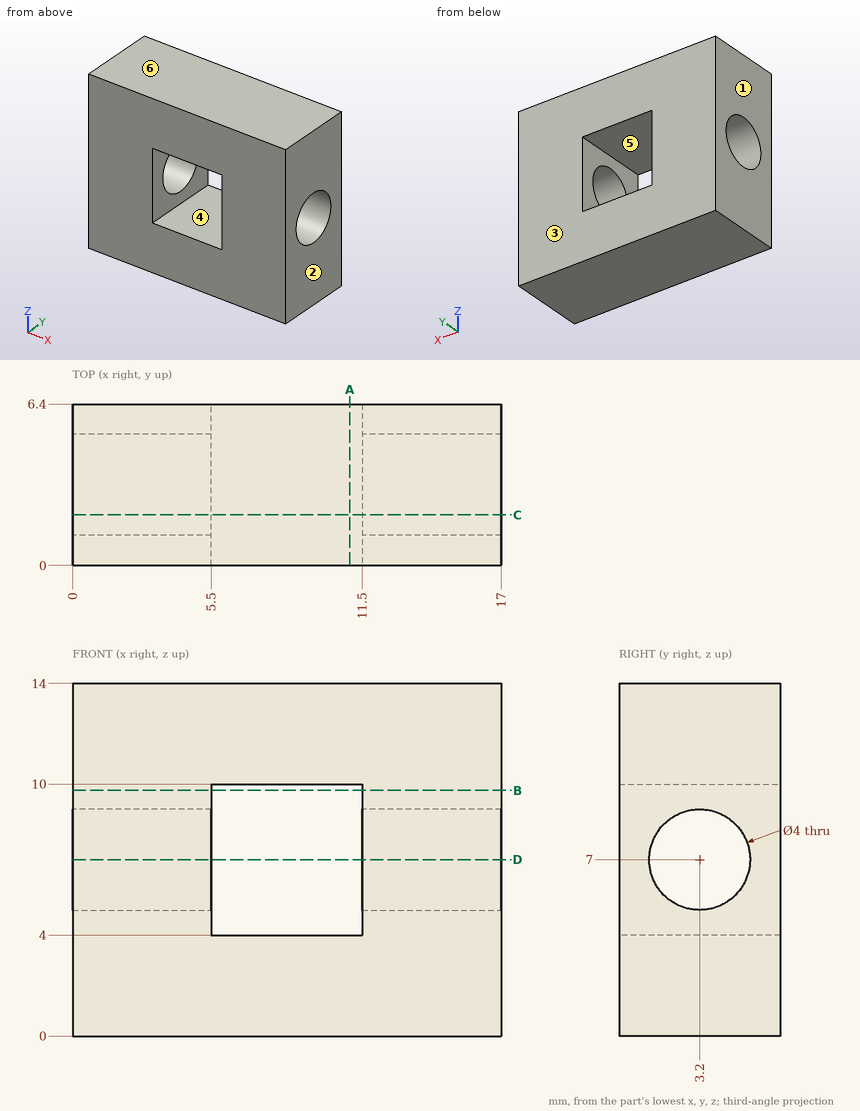
Job drawing, mm, ordinate dimensions from the low corner. One solid piece. A direction names the side the tool comes from. Coordinates: 2 decimals unless noted, no trailing zeros. Write each loop counter-clockwise with the first axis right and the second up, starting at its lowest first coordinate (ties: lowest second). Pieces come first, ordered by that corner, then holes.
Item 1: Slice it at B-B (z = 9.75). Write the cut outline in (x, y), and give its area (3 significant figures).
Item 2: Mould opens along X. For the marked faces 1, 2, 3 and 4 say: released by +X, released by -X, zero draft, split by the parting line, or undercut.
Item 3: Slice it at C-C (y = 2). Write the cut outline in (x, z).
Item 4: Probe line 1 (X direction, y = 5.5, z = 5); line 2 (Z direction, x = 8, y = 1.25); line 3 (Y direction, x = 1.4, z = 7). List the from-to ranges inside material, lowest first.
Item 5: Slice it at D-D (z = 7). Write the cut outline in (x, y), and give its area (3 significant figures).
Item 6: Pin check, flat tips, straight feed: pin 1 (1.8 mm diameter, centred on y = 1.5, z = 8, fed in from -X); pin 2 (3.5 mm diameter, centred on y = 3.2, z = 7, fed in from -X). Stop position of each tip, or through.
Item 7: Which spindle directions (+Z, -Z, +X, -X, +Y, -Y) get a long thin tool onto all of the face, cutting with end or side? Do the marked faces 5 and 6. Say none if no direction does.
Item 8: Slice it at A-A (x = 11). Write the cut outline in (y, z).
Results found:
1. outline: (0, 0) - (5.5, 0) - (5.5, 6.4) - (0, 6.4) - close; (11.5, 0) - (17, 0) - (17, 6.4) - (11.5, 6.4) - close
1. area: 70.4 mm2
2. face 1: released by -X
2. face 2: released by +X
2. face 3: zero draft
2. face 4: undercut
3. outline: (0, 0) - (17, 0) - (17, 5.4) - (11.5, 5.4) - (11.5, 4) - (5.5, 4) - (5.5, 5.4) - (0, 5.4) - close; (0, 8.6) - (5.5, 8.6) - (5.5, 10) - (11.5, 10) - (11.5, 8.6) - (17, 8.6) - (17, 14) - (0, 14) - close
4. line 1: x = 0 to 5.5, 11.5 to 17
4. line 2: z = 0 to 4, 10 to 14
4. line 3: y = 0 to 1.2, 5.2 to 6.4
5. outline: (0, 0) - (5.5, 0) - (5.5, 1.2) - (0, 1.2) - close; (0, 5.2) - (5.5, 5.2) - (5.5, 6.4) - (0, 6.4) - close; (11.5, 0) - (17, 0) - (17, 1.2) - (11.5, 1.2) - close; (11.5, 5.2) - (17, 5.2) - (17, 6.4) - (11.5, 6.4) - close
5. area: 26.4 mm2
6. pin 1: stops at x = 0
6. pin 2: passes through
7. face 5: +Y, -Y
7. face 6: +Z, +X, -X, +Y, -Y
8. outline: (0, 0) - (6.4, 0) - (6.4, 4) - (0, 4) - close; (0, 10) - (6.4, 10) - (6.4, 14) - (0, 14) - close
